```python
from build123d import *

# Parameters (mm, degrees)
F0_W      = 762
F0_H      = 762
F1_DEPTH  = 38.1
F2_W      = 76.2
F2_H      = 76.2
F3_DEPTH  = 609.6
F4_R      = 18.25625
F5_DEPTH  = 3.60934
F6_R      = 11.1125
F7_DEPTH  = 644.09166
F9_R      = 25.4
F9_R_2    = 23.8125
F10_DEPTH = 12.7
F11_W     = 127
F11_H     = 152.4
F12_DEPTH = 25.4


# Not quite as in the source:
# - a feature of the source that left no trace in its solid (it failed there, or was rolled back) is left out


with BuildPart() as f1:
    # F0 (on Top) → F1 (new body)
    with BuildSketch(Plane.XY):
        Rectangle(F0_W, F0_H)
    extrude(amount=F1_DEPTH)

    # F2 (on face) → F3 (join)
    with BuildSketch(Plane(origin=(0, 0, 0), x_dir=(1, 0, 0), z_dir=(0, 0, -1))):
        with Locations((-342.9, 342.9)):
            Rectangle(F2_W, F2_H)
        with Locations((342.9, 342.9)):
            Rectangle(F2_W, F2_H)
        with Locations((342.9, -342.9)):
            Rectangle(F2_W, F2_H)
        with Locations((-342.9, -342.9)):
            Rectangle(F2_W, F2_H)
    extrude(amount=F3_DEPTH)

    # F4 (on face) → F5 (cut)
    with BuildSketch(Plane.XY.offset(38.1)):
        Circle(F4_R)
    extrude(amount=-F5_DEPTH, mode=Mode.SUBTRACT)

    # F6 (on face) → F7 (cut, through all)
    with BuildSketch(Plane.XY.offset(34.49066)):
        Circle(F6_R)
    extrude(amount=-F7_DEPTH, mode=Mode.SUBTRACT)

    # F9 (on face) → F10 (cut)
    with BuildSketch(Plane.XY.offset(38.1)):
        Circle(F9_R)
        Circle(F9_R_2, mode=Mode.SUBTRACT)
    extrude(amount=-F10_DEPTH, mode=Mode.SUBTRACT)

    # F11 (on face) → F12 (join)
    with BuildSketch(Plane.XZ.offset(381)):
        with Locations((-241.3, -76.2)):
            Rectangle(F11_W, F11_H)
    extrude(amount=-F12_DEPTH)


solid = f1.part
```
The model under review builds one solid part; all positions refer to its coordinate system, in mm. A direction names the side the tool comes from. Give positions to 0.01 mm unless a question says otherwise; leave off trailing zeros. Write each loop counter-clockwise with the first axis right and the second up, starting at its lowest first coordinate (ties: lowest second). Pieces come first, ordered by that corner, then holes. Notation, with made-up numbers: (67, -35.75) -> (89, -35.75) arc R18 ccw to (89, -19.75) -> close; hole circle Ø10 at (-28.5, -24). An arc over 180 degrees is marked (long way). Answer in a Markdown table with one row per item.
1) Tool access review of faces 4 (the flat face through (-381, 86, 4)), 5 (the flat face through (-343, 304.8, -301)), 6 (the flat face through (304.8, -342, -301)), 7 (the flat face through (-304.8, 343, -301)), 8 (the cylindrical face through (-5.506, -24.796, 31.839)): name each direction out of +Z, -Z, +X, -X, +Y, -Y from which nothing blocks a thin tool from reaching the whole face with its end or side.
Worked answers:
| item | result |
|---|---|
| face 4 | +Z, -Z, -X, +Y, -Y |
| face 5 | -Z, +X, -X |
| face 6 | -Z, +Y, -Y |
| face 7 | -Z, +Y |
| face 8 | +Z |
2) Add section B-B on x = 0. State the section outline as (y, z) points.
Worked answers:
| item | result |
|---|---|
| outline | (-381, 0) -> (-11.11, 0) -> (-11.11, 34.49) -> (-18.26, 34.49) -> (-18.26, 38.1) -> (-23.81, 38.1) -> (-23.81, 25.4) -> (-25.4, 25.4) -> (-25.4, 38.1) -> (-381, 38.1) -> close; (11.11, 0) -> (381, 0) -> (381, 38.1) -> (25.4, 38.1) -> (25.4, 25.4) -> (23.81, 25.4) -> (23.81, 38.1) -> (18.26, 38.1) -> (18.26, 34.49) -> (11.11, 34.49) -> close |
3) Mouldability with a two-part tool opening along Y and no side actions: class faces 1 (the flat face through (-343, -304.8, -301)), 2 (the flat face through (-242, -355.6, -75)), 3 (the flat face through (-343, 342, -609.6)) as +Y half, -Y half, draft (parallel to the pull), parting line (faces both ways), or undercut.
Worked answers:
| item | result |
|---|---|
| face 1 | undercut |
| face 2 | +Y half |
| face 3 | draft |
4) Clearance check with flat-ended pins moving along their axes: P1, Ø12, axis at x = 68.5, y = 123, coming from the -Z side; P2, Ø11, axis at x = -8, y = -5.5, coming from the +Z side. State where each tip first meets the part, or that it passes through.
Worked answers:
| item | result |
|---|---|
| P1 | z = 0 |
| P2 | z = 34.49 |
5) Add section D-D on y = -205. State the section outline as (x, z) points, plus the area to 3 significant figures.
Worked answers:
| item | result |
|---|---|
| outline | (-381, 0) -> (381, 0) -> (381, 38.1) -> (-381, 38.1) -> close |
| area | 29,000 mm² |
6) Add section A-A on z = -277. State the section outline as (x, y) points.
Worked answers:
| item | result |
|---|---|
| outline | (-381, -381) -> (-304.8, -381) -> (-304.8, -304.8) -> (-381, -304.8) -> close; (-381, 304.8) -> (-304.8, 304.8) -> (-304.8, 381) -> (-381, 381) -> close; (304.8, -381) -> (381, -381) -> (381, -304.8) -> (304.8, -304.8) -> close; (304.8, 304.8) -> (381, 304.8) -> (381, 381) -> (304.8, 381) -> close |
7) For L1, parallel to Y at x = 0, z = 34; L2, parallel to X at y = -327, z = -4; L3, parallel to Y at x = 0, z = 10, list the stretches that pass through material, from the lowest coordinate up. Write a range as [from, to].
Worked answers:
| item | result |
|---|---|
| L1 | [-381, -25.4], [-23.81, -11.11], [11.11, 23.81], [25.4, 381] |
| L2 | [-381, -304.8], [304.8, 381] |
| L3 | [-381, -11.11], [11.11, 381] |
